Geometry: see drawing. Coordinates: mm, zero at the bounding-box minimum. A direction names the side the tool comes from. Give positions to 0.01 mm unless a question says otherwise; leave off trailing zeros. Order: outer loops, then holes, each group sorted by start corner. A loop starts at its lowest first (then second) coordinate and runs counter-clockwise, first axis right, second up. Notation, with made-up numbers: M 16.5,44 L 58.5,44 A14 ccw 58.5,59 Z; hole C 1.25,89.25 d7. An arc over 180 degrees is marked long. Write item = value, one per line. Start each with the question number.
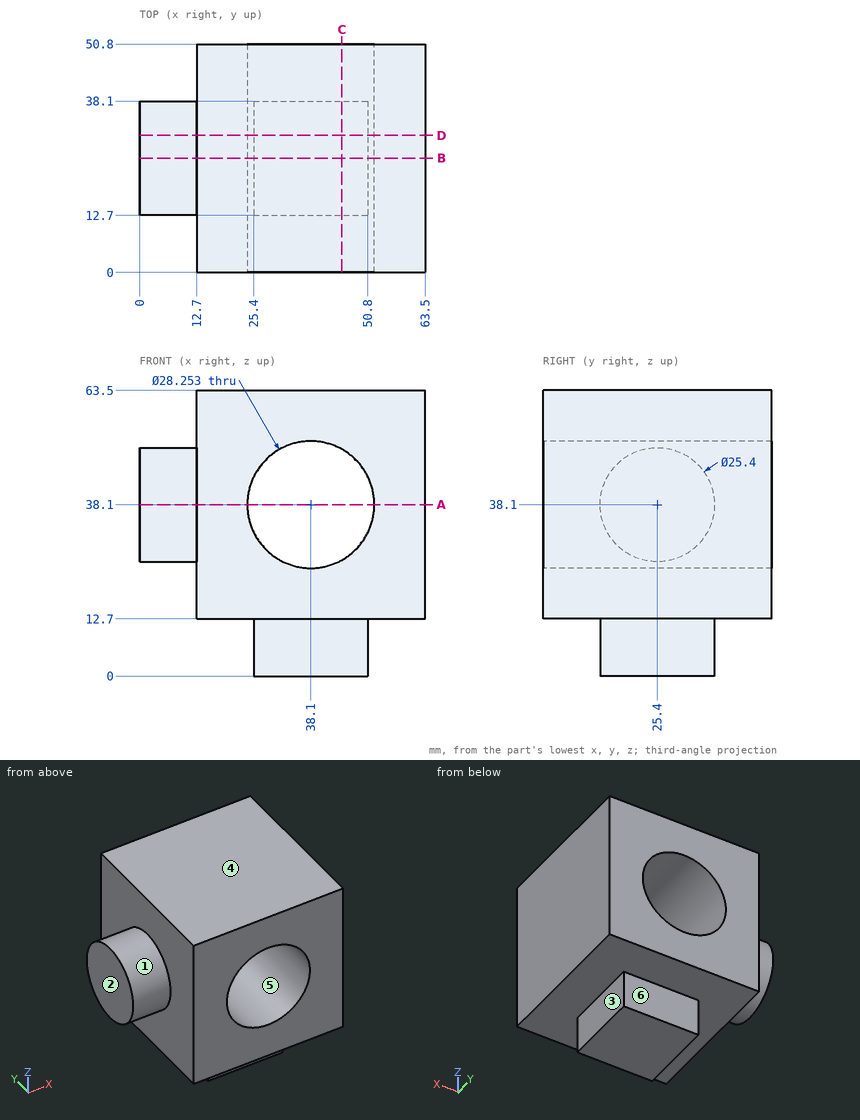
1) Cut plane C-C (x = 45). Return loops of the section in (y, z), plus the area to 3 significant figures.
2) Draft query along Z for the marked faces 4, 5 and 6. Return one class per face: pulls with the +Z half, pulls with the -Z half, needs draft (parallel to the pull), parting line crosses it, or undercut.
3) Cut plane D-D (y = 30.5). Return loops of the section in (x, z), plus the area to 3 significant figures.
4) Pin query (flat end, axial travel): pin 1 Ø10 at (x, z) = (44, 5) entering from +Y; pin 2 Ø4 at (x, z) = (33, 4.5) entering from -Y; pin 3 Ø14 at (y, z) = (27, 3.5) entering from -X. Return the tip coordinate at first contact, or that it passes through.
5) Ray query, L1, parallel to Z at x = 38.1, y = 38; L2, parallel to Z at x = 37.5, y = 47; L3, parallel to X at y = 38, z = 38 (1 decimal). Return the intervals inside material, ascending.
6) Access query for the marked faces 1, 2 and 3. Directions: +Z, -Z, +X, -X, +Y, -Y. A direction counts if a zero-diameter tool reaches every point of the face in a straight line with its end or side. Return the directions, or none.
7) Cut plane B-B (y = 25.4). Return loops of the section in (x, z).
8) Cut plane A-A (z = 38.1). Return loops of the section in (x, y).
Reply:
q1.outline = M 0,12.7 L 12.7,12.7 L 12.7,0 L 38.1,0 L 38.1,12.7 L 50.8,12.7 L 50.8,25.77 L 0,25.77 Z; M 0,50.43 L 50.8,50.43 L 50.8,63.5 L 0,63.5 Z
q1.area = 1,650 mm²
q2.face_4 = pulls with the +Z half
q2.face_5 = undercut
q2.face_6 = needs draft
q3.outline = M 0,26.47 L 12.7,26.47 L 12.7,12.7 L 25.4,12.7 L 25.4,0 L 50.8,0 L 50.8,12.7 L 63.5,12.7 L 63.5,63.5 L 12.7,63.5 L 12.7,49.73 L 0,49.73 Z; hole C 38.1,38.1 d28.25
q3.area = 2,570 mm²
q4.pin_1 = 38.1
q4.pin_2 = 12.7
q4.pin_3 = 25.4
q5.L1 = 0 to 23.97, 52.23 to 63.5
q5.L2 = 12.7 to 23.99, 52.21 to 63.5
q5.L3 = 0 to 24, 52.2 to 63.5
q6.face_1 = -X
q6.face_2 = +Z, -Z, -X, +Y, -Y
q6.face_3 = -Z, +X, +Y, -Y
q7.outline = M 0,25.4 L 12.7,25.4 L 12.7,12.7 L 25.4,12.7 L 25.4,0 L 50.8,0 L 50.8,12.7 L 63.5,12.7 L 63.5,63.5 L 12.7,63.5 L 12.7,50.8 L 0,50.8 Z; hole C 38.1,38.1 d28.25
q8.outline = M 0,12.7 L 12.7,12.7 L 12.7,0 L 23.97,0 L 23.97,50.8 L 12.7,50.8 L 12.7,38.1 L 0,38.1 Z; M 52.23,0 L 63.5,0 L 63.5,50.8 L 52.23,50.8 Z
